Verification items for the finished model (mm, model axes). Round coordinates to 2 decimals unless told otherwise and drop trailing zeros. Write each loop counter-clockwise with the first axis right and the second up, starting at its lowest first coordinate (ties: lowest second). Pieces come first, ordered by that corner, then holes. Notation, with made-up numbers: (35.25, 58.5) - (45.25, 58.5) arc R29 cw to (45.25, 95.5) - close; hole circle Ø10 at (31.25, 89). An arc over 180 degrees is marked (long way). Write each question's results on one line, items separated by ' | '.
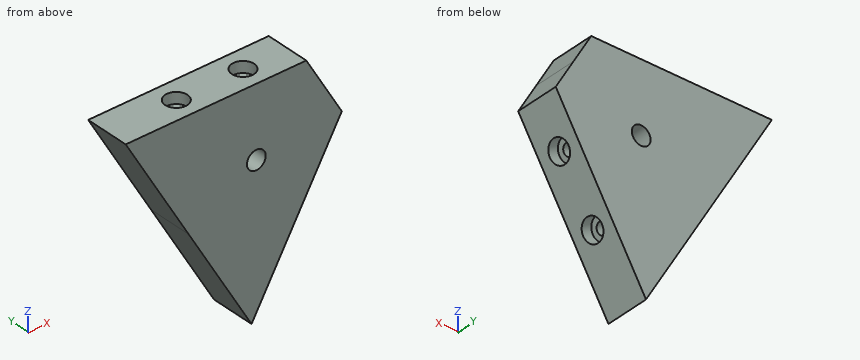
```python
from build123d import *

# Parameters (mm, degrees)
BOSS_EXTRUDE1_DEPTH = 25.4
SKETCH2_R           = 6.35
CUT_EXTRUDE1_DEPTH  = 6.35
SKETCH3_R           = 3.2639
CUT_EXTRUDE2_DEPTH  = 16.51
SKETCH4_R           = 3.2639
CUT_EXTRUDE3_DEPTH  = 16.51
SKETCH5_R           = 5.3578125
CUT_EXTRUDE4_DEPTH  = 280.690442894


with BuildPart() as part:
    # Sketch1 → Boss-Extrude1 (new body)
    with BuildSketch(Plane(origin=(0, 0, 0), x_dir=(1, 0, 0), z_dir=(0, 1, 0))):
        Polygon((119.068292428, -241.162389864), (129.21607637, -223.585912492), (51.895065274, -178.944605922), (15.973610966, -241.162389864), align=None)
    boss_extrude1 = extrude(amount=BOSS_EXTRUDE1_DEPTH)

    # Sketch2 → Cut-Extrude1 (cut)
    with BuildSketch(Plane.XY.offset(241.162389864)):
        with Locations((55.568292428, 12.7)):
            Circle(SKETCH2_R)
        with Locations((93.668292428, 12.7)):
            Circle(SKETCH2_R)
    cut_extrude1 = extrude(amount=-CUT_EXTRUDE1_DEPTH, mode=Mode.SUBTRACT)

    # Sketch3 → Cut-Extrude2 (cut)
    with BuildSketch(Plane.XY.offset(234.812389864)):
        with Locations((55.568292428, 12.7)):
            Circle(SKETCH3_R)
    cut_extrude2 = extrude(amount=-CUT_EXTRUDE2_DEPTH, mode=Mode.SUBTRACT)

    # Sketch4 → Cut-Extrude3 (cut)
    with BuildSketch(Plane.XY.offset(234.812389864)):
        with Locations((93.668292428, 12.7)):
            Circle(SKETCH4_R)
    cut_extrude3 = extrude(amount=-CUT_EXTRUDE3_DEPTH, mode=Mode.SUBTRACT)

    # Mirror1: Boss-Extrude1, Cut-Extrude1, Cut-Extrude2, Cut-Extrude3 across plane
    add(boss_extrude1.mirror(Plane(origin=(51.895065274, 25.4, 178.944605922), x_dir=(0.8660254037844389, 0, 0.4999999999999996), z_dir=(-0.49999999999999983, 0, 0.8660254037844388))))
    add(cut_extrude1.mirror(Plane(origin=(51.895065274, 25.4, 178.944605922), x_dir=(0.8660254037844389, 0, 0.4999999999999996), z_dir=(-0.49999999999999983, 0, 0.8660254037844388))), mode=Mode.SUBTRACT)
    add(cut_extrude2.mirror(Plane(origin=(51.895065274, 25.4, 178.944605922), x_dir=(0.8660254037844389, 0, 0.4999999999999996), z_dir=(-0.49999999999999983, 0, 0.8660254037844388))), mode=Mode.SUBTRACT)
    add(cut_extrude3.mirror(Plane(origin=(51.895065274, 25.4, 178.944605922), x_dir=(0.8660254037844389, 0, 0.4999999999999996), z_dir=(-0.49999999999999983, 0, 0.8660254037844388))), mode=Mode.SUBTRACT)

    # Sketch5 → Cut-Extrude4 (cut, through all)
    with BuildSketch(Plane(origin=(0, 25.4, 0), x_dir=(1, 0, 0), z_dir=(0, 1, 0))):
        with Locations(Location((90.555570822, -201.265259207, 0), (0, 0, 270))):
            Circle(SKETCH5_R)
    extrude(amount=-CUT_EXTRUDE4_DEPTH, mode=Mode.SUBTRACT)


solid = part.part
```
(1) Thickness scan on L1, parallel to Z at x = 90.5, y = 14; L2, parallel to Y at x = 105.5, z = 153; L3, parallel to Z at x = 92, y = 10. Record the ranges inside material, lowest first.
Answer:
L1: 121.37 to 157.44, 164.35 to 195.91, 206.62 to 234.81 | L2: 0 to 6.38, 19.02 to 25.4 | L3: 123.97 to 157.91, 162.15 to 196.11, 206.42 to 218.3
(2) Section check C-C (x = 55.5). Record the cut outline in (y, z), plus the area to 3 significant figures.
Answer:
outline: (0, 172.7) - (25.4, 172.7) - (25.4, 241.16) - (19.05, 241.16) - (19.05, 234.81) - (15.96, 234.81) - (15.96, 218.3) - (9.44, 218.3) - (9.44, 234.81) - (6.35, 234.81) - (6.35, 241.16) - (0, 241.16) - close | area: 1,550 mm2
(3) Section check D-D (z = 231.5). Record the cut outline in (x, y), plus the area to 3 significant figures.
Answer:
outline: (21.55, 0) - (124.65, 0) - (124.65, 25.4) - (21.55, 25.4) - close; hole circle Ø6.53 at (55.57, 12.7); hole circle Ø6.53 at (93.67, 12.7) | area: 2,550 mm2
(4) Section check A-A (z = 203). Record the cut outline in (x, y).
Answer:
outline: (38.01, 0) - (85.49, 0) - (85.49, 25.4) - (38.01, 25.4) - close; (95.62, 0) - (137.63, 0) - (137.63, 25.4) - (95.62, 25.4) - close
(5) Section check B-B (y = 2.25). Record the cut outline in (x, z).
Answer:
outline: (15.97, 241.16) - (87.82, 116.73) - (139.36, 206.01) - (119.07, 241.16) - close; hole circle Ø10.72 at (90.56, 201.27)
(6) Go/stop test with flat-tipped pins: pin 1 Ø1 at (y, z) = (21.5, 132.5) entering from +X; pin 2 Ø8 at (x, y) = (123.5, 7) entering from -Z; pin 3 Ø3.5 at (x, y) = (54.5, 12.5) entering from +Z. Record where each tip stops, or that it passes through.
Answer:
pin 1: x = 97.21 | pin 2: z = 171.6 | pin 3: z = 218.3
